Source: CAD feature listing. Evaluate the final solid. Frame: model axes, mm. Give positions to 0.01 mm unless a question says otherwise; leave off trailing zeros. Order: outer loops, then holes, each group sorted by start corner. A loop starts at its lowest first (then second) coordinate and runs counter-clockwise, first axis right, second up. Notation, with made-up numbers: M 67.25,42.25 L 105.25,42.25 A27 ccw 105.25,65.25 Z; hole C -4.75,-33.5 d3. An arc over 180 degrees is marked long. One line per question, with ' | ' between items. Start each with the question number.
from build123d import *

# Parameters (mm, degrees)
BOSS_EXTRUDE1_DEPTH = 5


with BuildPart() as part:
    # Sketch1 → Boss-Extrude1 (new body, symmetric)
    with BuildSketch(Plane.XY):
        with BuildLine():
            Line((-11.5, -54.47), (-135, -54.47))
            Line((-135, -54.47), (-135, 44.47))
            Line((-135, 44.47), (135, 44.47))
            Line((135, 44.47), (135, -54.47))
            Line((135, -54.47), (11.5, -54.47))
            ThreePointArc((11.5, -54.47), (0, -42.97), (-11.5, -54.47))
        make_face()
    extrude(amount=BOSS_EXTRUDE1_DEPTH, both=True)


solid = part.part
Item 1: Mould query, pull axis X, two halves, no side actions, for faces 1 (the flat face through (135, -4, 0)), 2 (the flat face through (2, -4, 5)), 3 (the flat face through (-135, -6, 0)), 4 (the cylindrical face through (0.253, -42.973, 0.07)). Classes: pulls with the +X half, pulls with the -X half, needs draft (parallel to the pull), parting line crosses it, or undercut.
Item 2: Cut plane A-A on x = 0. Return the cut outline in (y, z), and give its area (3 significant figures).
Item 3: Line query: line 1 (X direction, y = -50, z = -2); line 2 (Y direction, x = 7, z = -0.5). Output: solid intervals per line, ascending.
Results are:
1) face 1: pulls with the +X half | face 2: needs draft | face 3: pulls with the -X half | face 4: undercut
2) outline: M -42.97,-5 L 44.47,-5 L 44.47,5 L -42.97,5 Z | area: 874 mm2
3) line 1: x = -135 to -10.6, 10.6 to 135 | line 2: y = -45.35 to 44.47
